Part model, mm, in its own coordinate system. A direction names the side the tool comes from. Round coordinates to 2 decimals unless told otherwise and drop trailing zeros. Loops run counter-clockwise (first coordinate to the right, second up) from the corner with the lowest first, then second, coordinate; pieces in that order, holes last.
from build123d import *

# Parameters (mm, degrees)
SKETCH1_W           = 60
SKETCH1_H           = 60
BOSS_EXTRUDE1_DEPTH = 15
FILLET1_R           = 3
SHELL1_START        = -27
SHELL1_OUTLINE_W    = 12
SHELL1_OUTLINE_H    = 54
SHELL1_DEPTH        = 54


# Read off the part's stored shape, not the designer's step: Shell1
with BuildPart() as part:
    # Sketch1 → Boss-Extrude1 (new body)
    with BuildSketch(Plane(origin=(0, 0, 0), x_dir=(1, 0, 0), z_dir=(0, 1, 0))):
        Rectangle(SKETCH1_W, SKETCH1_H)
    extrude(amount=BOSS_EXTRUDE1_DEPTH)

    # Fillet1
    fillet1_edges = [part.edges().sort_by_distance(p)[0] for p in [
        (30, 15, 0),
        (0, 15, -30),
        (-30, 15, 0),
        (0, 15, 30),
        (-30, 7.5, -30),
        (30, 7.5, -30),
        (30, 7.5, 30),
        (-30, 7.5, 30),
    ]]
    fillet(fillet1_edges, radius=FILLET1_R)

    # Shell1 outline → Shell1 (cut)
    with BuildSketch(Plane.YZ.offset(SHELL1_START)):
        with Locations((6, 0)):
            Rectangle(SHELL1_OUTLINE_W, SHELL1_OUTLINE_H)
    extrude(amount=SHELL1_DEPTH, mode=Mode.SUBTRACT)


solid = part.part
1) Slice it at C-C, the plane x = 5. Give the cut face in (y, z).
Values:
outline: (0, -30) - (12, -30) arc R3 ccw to (15, -27) - (15, 27) arc R3 ccw to (12, 30) - (0, 30) - (0, 27) - (12, 27) - (12, -27) - (0, -27) - close
2) Wall check: line 1 along Z through (x, y) = (-5, 2.75); line 2 along Y through (x, z) = (2, -4). Give the ranges that are in metal, low to high.
Values:
line 1: z = -30 to -27, 27 to 30
line 2: y = 12 to 15
3) Drop a flat-ended pin along its axis: pin 1 Ø1 at (x, z) = (-1, -15) entering from -Y. Give the stop position or say it passes through.
Values:
pin 1: stops at y = 12
4) Mould opens along X. For faces 3 (the face through (29.14, 6.08, -29.1)), 4 (the face through (-27, 6, 0)), 5 (the face through (0.38, 14.1, 29.14)) say: released by +X, released by -X, zero draft, split by the parting line, or undercut.
Values:
face 3: released by +X
face 4: undercut
face 5: zero draft
5) Slice it at A-A, the plane z = -2.5. Give the cut face in (x, y).
Values:
outline: (-30, 0) - (-27, 0) - (-27, 12) - (27, 12) - (27, 0) - (30, 0) - (30, 12) arc R3 ccw to (27, 15) - (-27, 15) arc R3 ccw to (-30, 12) - close
6) Tool access for faces 1 (the face through (27, 6, 0)), 2 (the face through (30, 6, 0)): list every direction of +Z, -Z, +X, -X, +Y, -Y with a clear straight run to the whole face (end or side of a thin tool).
Values:
face 1: -Y
face 2: +Z, -Z, +X, +Y, -Y
7) Slice it at B-B, the plane y = 4.5. Give the cut face in (x, z), then the cut area to 3 significant figures.
Values:
outline: (-30, -27) arc R3 ccw to (-27, -30) - (27, -30) arc R3 ccw to (30, -27) - (30, 27) arc R3 ccw to (27, 30) - (-27, 30) arc R3 ccw to (-30, 27) - close; hole (-27, -27) - (27, -27) - (27, 27) - (-27, 27) - close
area: 676 mm2
